```python
from build123d import *

# Parameters (mm, degrees)
BOSS_EXTRUDE1_DEPTH = 3.175
MIRROR1_OUTLINE_W   = 3.175
MIRROR1_OUTLINE_H   = 6.35
MIRROR1_DEPTH       = 248.225
MIRROR1_2_OUTLINE_W = 3.175
MIRROR1_2_OUTLINE_H = 116.175
MIRROR1_2_DEPTH     = 6.35
MIRROR1_START       = 84.858333333
MIRROR1_3_OUTLINE_W = 3.175
MIRROR1_3_OUTLINE_H = 6.35
MIRROR1_3_DEPTH     = 75.333333334
MIRROR1_START_2     = 6.35
MIRROR1_4_OUTLINE_W = 3.175
MIRROR1_4_OUTLINE_H = 34.491666667
MIRROR1_4_DEPTH     = 6.35
MIRROR1_START_3     = 241.875
MIRROR1_5_OUTLINE_W = 3.175
MIRROR1_5_OUTLINE_H = 6.35
MIRROR1_5_DEPTH     = 6.35
MIRROR1_START_4     = 238.7
MIRROR1_6_OUTLINE_W = 3.175
MIRROR1_6_OUTLINE_H = 2.116666666
MIRROR1_6_DEPTH     = 3.175
SKETCH2_W           = 3.175
SKETCH2_H           = 3.175
CUT_EXTRUDE1_DEPTH  = 3.175


# Read off the part's stored shape, not the designer's step: Mirror1
with BuildPart() as part:
    # Sketch1 → Boss-Extrude1 (new body)
    with BuildSketch(Plane(origin=(0, 0, 0), x_dir=(0, 0, -1), z_dir=(1, 0, 0))):
        Polygon((6.35, 232.35), (0, 232.35), (0, 0), (122.525, 0), (122.525, 12.7), (88.033333333, 12.7), (88.033333333, 6.35), (6.35, 6.35), (6.35, 84.858333333), (12.7, 84.858333333), (12.7, 160.191666667), (6.35, 160.191666667), align=None)
        Polygon((-2.116666667, 241.875), (0, 241.875), (0, 232.35), (6.35, 232.35), (6.35, 248.225), (-6.35, 248.225), (-6.35, 241.875), (-4.233333333, 241.875), (-4.233333333, 238.7), (-2.116666667, 238.7), align=None)
    extrude(amount=BOSS_EXTRUDE1_DEPTH)



with BuildPart() as body_2:
    # Mirror1 outline → Mirror1 (new body)
    with BuildSketch(Plane(origin=(0, 0, 0), x_dir=(1, 0, 0), z_dir=(0, 1, 0))):
        with Locations((1.5875, 241.875)):
            Rectangle(MIRROR1_OUTLINE_W, MIRROR1_OUTLINE_H)
    extrude(amount=MIRROR1_DEPTH)


with BuildPart() as part_1:
    add(part.part)

    add(body_2.part)  # Mirror1 2 merges body 2
    # Mirror1 2 outline → Mirror1 2 (add)
    with BuildSketch(Plane(origin=(0, 0, 0), x_dir=(1, 0, 0), z_dir=(0, 1, 0))):
        with Locations((1.5875, 180.6125)):
            Rectangle(MIRROR1_2_OUTLINE_W, MIRROR1_2_OUTLINE_H)
    extrude(amount=MIRROR1_2_DEPTH)

    # Mirror1 3 outline → Mirror1 3 (add)
    with BuildSketch(Plane(origin=(0, 0, 0), x_dir=(1, 0, 0), z_dir=(0, 1, 0)).offset(MIRROR1_START)):
        with Locations((1.5875, 235.525)):
            Rectangle(MIRROR1_3_OUTLINE_W, MIRROR1_3_OUTLINE_H)
    extrude(amount=MIRROR1_3_DEPTH)

    # Mirror1 4 outline → Mirror1 4 (add)
    with BuildSketch(Plane(origin=(0, 0, 0), x_dir=(1, 0, 0), z_dir=(0, 1, 0)).offset(MIRROR1_START_2)):
        with Locations((1.5875, 139.770833334)):
            Rectangle(MIRROR1_4_OUTLINE_W, MIRROR1_4_OUTLINE_H)
    extrude(amount=MIRROR1_4_DEPTH)

    # Mirror1 5 outline → Mirror1 5 (add)
    with BuildSketch(Plane(origin=(0, 0, 0), x_dir=(1, 0, 0), z_dir=(0, 1, 0)).offset(MIRROR1_START_3)):
        with Locations((1.5875, 248.225)):
            Rectangle(MIRROR1_5_OUTLINE_W, MIRROR1_5_OUTLINE_H)
    extrude(amount=MIRROR1_5_DEPTH)

    # Mirror1 6 outline → Mirror1 6 (add)
    with BuildSketch(Plane(origin=(0, 0, 0), x_dir=(1, 0, 0), z_dir=(0, 1, 0)).offset(MIRROR1_START_4)):
        with Locations((1.5875, 248.225)):
            Rectangle(MIRROR1_6_OUTLINE_W, MIRROR1_6_OUTLINE_H)
    extrude(amount=MIRROR1_6_DEPTH)

    # Sketch2 → Cut-Extrude1 (cut)
    with BuildSketch(Plane(origin=(3.175, 0, 0), x_dir=(0, 0, -1), z_dir=(1, 0, 0))):
        with Locations((83.270833333, 1.5875)):
            Rectangle(SKETCH2_W, SKETCH2_H)
        with Locations((161.779166667, 4.7625)):
            Rectangle(SKETCH2_W, SKETCH2_H)
    extrude(amount=-CUT_EXTRUDE1_DEPTH, mode=Mode.SUBTRACT)


solid = part_1.part
```
Verification items for the finished model (mm, model axes). Give positions to 0.01 mm unless a question says otherwise; leave off trailing zeros. Order: outer loops, then holes, each group sorted by start corner. A loop starts at its lowest first (then second) coordinate and runs counter-clockwise, first axis right, second up. Notation, with made-up numbers: M 85.5,69.25 L 144.5,69.25 A10 ccw 144.5,77.25 Z; hole C 77.5,-33 d6. An arc over 180 degrees is marked long. Return JSON: item names as keys, results as strings. Group by question number.
1) Section check C-C on z = -125. Record the cut outline in (x, y) (3 decimals), and give its area (3 significant figures).
2) Go/stop test with flat-tipped pins: pin 1 Ø1 at (x, y) = (1.5, 43.5) entering from -Z; pin 2 Ø1 at (x, z) = (2, -162) entering from +Y (3 decimals); pin 3 Ø0.6 at (x, z) = (2, -248) entering from -Y. Record where each tip stops, or that it passes through.
3) Scan lines: line 1 (Z direction, x = 2.45, y = 12.5); line 2 (Z direction, x = 2.85, y = 113.5); line 3 (Z direction, x = 2.65, y = 228). Record each from-to range of solid material in increasing order.
4) Section check D-D on z = -26. Record the cut outline in (x, y) (3 decimals).
5) Section check B-B on y = 113.5. Record the cut outline in (x, z) (3 decimals).
6) Section check A-A on y = 71. Record the cut outline in (x, z) (3 decimals).
Answer block:
{
 "1": {"outline": "M 0,0 L 3.175,0 L 3.175,12.7 L 0,12.7 Z", "area": "40.3 mm^2"},
 "2": {"pin 1": "stops at z = -245.05", "pin 2": "stops at y = 3.175", "pin 3": "stops at y = 238.7"},
 "3": {"line 1": "z = -245.05 to -238.7, -157.02 to -88.03, -6.35 to 0", "line 2": "z = -245.05 to -232.35, -12.7 to 0", "line 3": "z = -245.05 to -238.7, -6.35 to 0"},
 "4": {"outline": "M 0,0 L 3.175,0 L 3.175,6.35 L 0,6.35 Z"},
 "5": {"outline": "M 0,-245.05 L 3.175,-245.05 L 3.175,-232.35 L 0,-232.35 Z; M 0,-12.7 L 3.175,-12.7 L 3.175,0 L 0,0 Z"},
 "6": {"outline": "M 0,-245.05 L 3.175,-245.05 L 3.175,-238.7 L 0,-238.7 Z; M 0,-6.35 L 3.175,-6.35 L 3.175,0 L 0,0 Z"}
}
